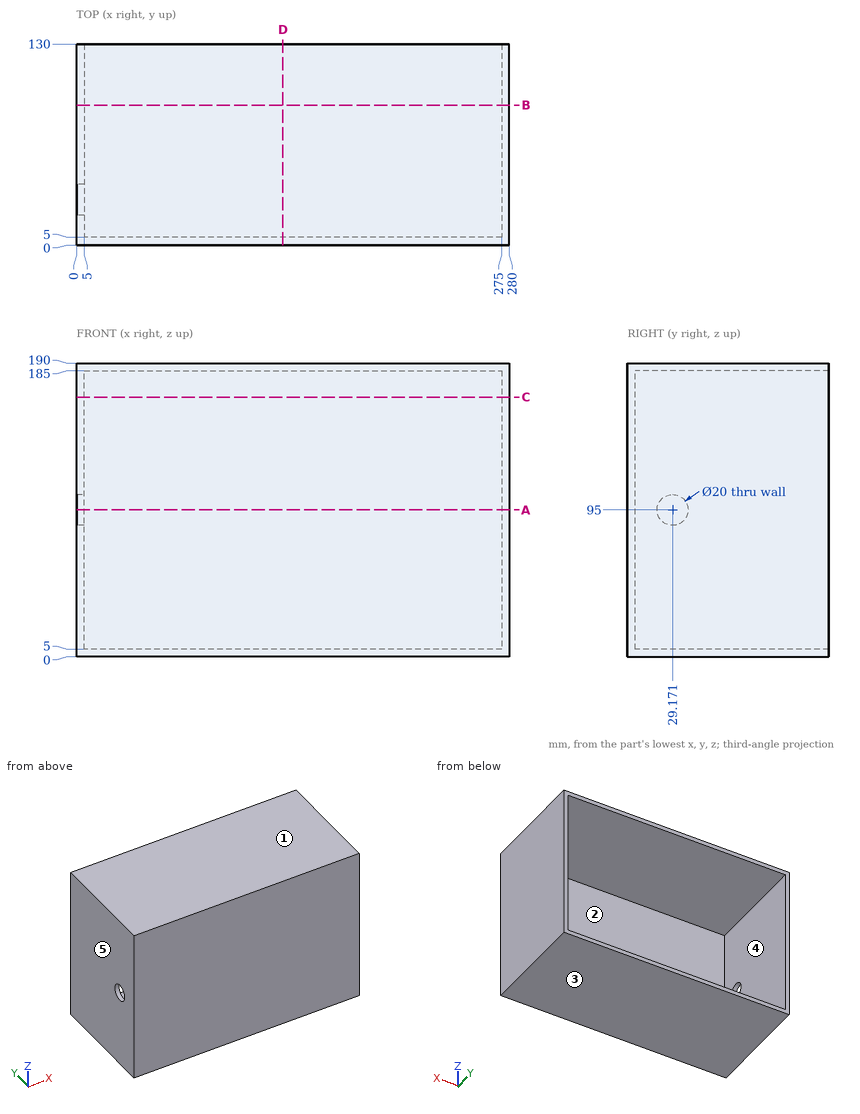
Input: dimensioned drawing with shaded views. Units: mm. Origin: part minimum x, y, z. A direction names the side the tool comes from. Round coordinates to 2 decimals unless told otherwise and drop trailing zeros. Write each loop counter-clockwise with the first axis right and the second up, starting at its lowest first coordinate (ties: lowest second). Pieces come first, ordered by that corner, then holes. Notation, with made-up numbers: (69, 58) -> (105, 58) arc R30 ccw to (105, 93) -> close; hole circle Ø5 at (16, 85.25). An arc over 180 degrees is marked (long way). Use CSV: the item, a comma, the result in double quotes. Start each with the question number.
Q1. Section D-D (x = 133.5). Return loops of the section in (y, z), plus the area to 3 significant figures.
Q2. Line query: L1, parallel to X at y = 121, z = 132; L2, parallel to Z at x = 139, y = 37; L3, parallel to Y at x = 3.85, z = 95. Output: solid intervals per line, ascending.
Q3. Pull-direction query (Z, two-part tool) for the marked faces 3, 4 and 5; classes: pulls with the +Z half, pulls with the -Z half, needs draft (parallel to the pull), parting line crosses it, or undercut.
Q4. Section A-A (z = 95). Return loops of the section in (x, y), plus the area to 3 significant figures.
Q5. Section B-B (y = 90.5). Return loops of the section in (x, z), plus the area to 3 significant figures.
Q6. Reachability of the marked faces 1 and 2 from +Z, -Z, +X, -X, +Y, -Y: full face, straight path, thin tool, end or side. Return the list, or none.
Q7. Section C-C (z = 168). Return loops of the section in (x, y), plus the area to 3 significant figures.
Q8. First-contact query: pin 1 Ø3 at (x, z) = (42.5, 167) entering from +Y. Flat tip, straight axial feed; report the tip coordinate or a pass-through.
Result sheet:
1,outline,"(0, 0) -> (130, 0) -> (130, 5) -> (5, 5) -> (5, 185) -> (130, 185) -> (130, 190) -> (0, 190) -> close"
1,area,"2,200 mm²"
2,L1,"0 to 5, 275 to 280"
2,L2,"0 to 5, 185 to 190"
2,L3,"0 to 19.17, 39.17 to 130"
3,face 3,"pulls with the -Z half"
3,face 4,"undercut"
3,face 5,"needs draft"
4,outline,"(0, 0) -> (280, 0) -> (280, 130) -> (275, 130) -> (275, 5) -> (5, 5) -> (5, 19.17) -> (0, 19.17) -> close; (0, 39.17) -> (5, 39.17) -> (5, 130) -> (0, 130) -> close"
4,area,"2,550 mm²"
5,outline,"(0, 0) -> (280, 0) -> (280, 190) -> (0, 190) -> close; hole (5, 5) -> (275, 5) -> (275, 185) -> (5, 185) -> close"
5,area,"4,600 mm²"
6,face 1,"+Z, +X, -X, +Y, -Y"
6,face 2,"+Y"
7,outline,"(0, 0) -> (280, 0) -> (280, 130) -> (275, 130) -> (275, 5) -> (5, 5) -> (5, 130) -> (0, 130) -> close"
7,area,"2,650 mm²"
8,pin 1,"y = 5"
